Read the model definition and answer for the solid it produces. Units are mm, in the model's axes. A direction names the side the tool comes from. Coordinates: 2 decimals unless noted, no trailing zeros. Write each loop counter-clockwise with the first axis right and the second up, starting at its lowest first coordinate (ties: lowest second). Pieces come first, ordered by that corner, then holes.
1) Which of the six approach directions +Z, -Z, +X, -X, +Y, -Y give full straight-line access (tool end or side, diameter ignored) to faces 1 (the face through (23.368, 18, 0)), 2 (the face through (-18, 23.368, 18)), 3 (the face through (19.8, 9.6, -20.51)), 4 (the face through (15.174, 18.139, -14.999))?
2) The part is cut by section A-A (y = 9.5). Determine the outline of the cut face in (x, z), then the cut area to 3 significant figures.
3) Each of these flat-tipped pins is pushed along its axis until it touches: pin 1 Ø2 at (x, z) = (16, -19.5) entering from -Y; pin 2 Ø3.5 at (x, y) = (27.5, 22.5) entering from -Z; pin 3 Ø2 at (y, z) = (17.5, 13) entering from +X. Where does it stop, or does it pass through?
4) The part is cut by section C-C (y = 18). Determine the outline of the cut face in (x, z).
5) Find the intervals of material crossed by line 1 (Y direction, x = 1.5, z = 17.5) (3 decimals); line 2 (X direction, y = 30, z = -8.5); line 3 (Y direction, x = -20.5, z = -3.5) (3 decimals), in increasing order.
6) The part is cut by section B-B (z = 0). Determine the outline of the cut face in (x, y) (3 decimals), then the cut area to 3 significant figures.
7) The part is cut by section D-D (x = 7.5). Determine the outline of the cut face in (y, z) (3 decimals).
8) Determine the mould class of faces 5 (the face through (16, 20.32, -17.3)), 6 (the face through (-16.62, 8.52, 16.43)), 7 (the face through (16.34, 12.81, -18.98)) for opening direction X: +X half, -X half, draft (parallel to the pull), parting line (faces both ways), or undercut.
from build123d import *

# Parameters (mm, degrees)
BOSS_EXTRUDE1_DEPTH  = 35.56
SHELL1_T             = -2.032
SKETCH2_R            = 15.24
BOSS_EXTRUDE2_DEPTH  = 3.175
SKETCH3_R            = 4.064
BOSS_EXTRUDE3_DEPTH  = 2.8575
FILLET2_R            = 2.54
SKETCH4_R            = 4.064
BOSS_EXTRUDE10_DEPTH = 2.8575
BOSS_EXTRUDE11_DEPTH = 8.636
FILLET3_R            = 2.54
BOSS_EXTRUDE12_DEPTH = 46.736
SKETCH8_W            = 5.08
SKETCH8_H            = 22.86
CUT_EXTRUDE1_DEPTH   = 55.98528445


with BuildPart() as part:
    # Sketch1 → Boss-Extrude1 (new body)
    with BuildSketch(Plane(origin=(0, 0, 0), x_dir=(1, 0, 0), z_dir=(0, 1, 0))):
        Polygon((9.679342526, -23.368), (23.368, -9.679342526), (23.368, 9.679342526), (9.679342526, 23.368), (-9.679342526, 23.368), (-23.368, 9.679342526), (-23.368, -9.679342526), (-9.679342526, -23.368), align=None)
    extrude(amount=BOSS_EXTRUDE1_DEPTH)

    # Shell1
    shell1_openings = [part.faces().sort_by_distance(p)[0] for p in [
        (0, 0, 0),
    ]]
    offset(amount=SHELL1_T, openings=shell1_openings, kind=Kind.INTERSECTION)

    # Sketch2 → Boss-Extrude2 (add)
    with BuildSketch(Plane.XZ):
        Polygon((23.368, 9.679342526), (9.679342526, 23.368), (-9.679342526, 23.368), (-23.368, 9.679342526), (-23.368, -9.679342526), (-9.679342526, -23.368), (9.679342526, -23.368), (23.368, -9.679342526), align=None)
        with Locations(Location((0, 0, 0), (0, 0, 270))):
            Circle(SKETCH2_R, mode=Mode.SUBTRACT)
    extrude(amount=-BOSS_EXTRUDE2_DEPTH)

    # Sketch3 → Boss-Extrude3 (add)
    with BuildSketch(Plane(origin=(0, 0, -23.368), x_dir=(-1, 0, 0), z_dir=(0, 0, -1))):
        with BuildLine():
            Line((-9.679342526, 5.08), (-27.205342526, 5.08))
            ThreePointArc((-27.205342526, 5.08), (-34.825342526, 12.7), (-27.205342526, 20.32))
            Line((-27.205342526, 20.32), (-9.679342526, 20.32))
            Line((-9.679342526, 20.32), (-9.679342526, 5.08))
        make_face()
        with Locations((-27.205342526, 12.7)):
            Circle(SKETCH3_R, mode=Mode.SUBTRACT)
    extrude(amount=-BOSS_EXTRUDE3_DEPTH)

    # Fillet2
    fillet2_edges = [part.edges().sort_by_distance(p)[0] for p in [
        (12.536842526, 12.7, -20.5105),
    ]]
    fillet(fillet2_edges, radius=FILLET2_R)

    # Sketch4 → Boss-Extrude10 (add)
    with BuildSketch(Plane.XY.offset(-20.5105)):
        with BuildLine():
            Line((12.981342526, 19.304), (12.981342526, 29.464))
            Line((12.981342526, 29.464), (24.665342526, 29.464))
            Line((24.665342526, 29.464), (33.422629122, 17.105649484))
            ThreePointArc((33.422629122, 17.105649484), (29.517124969, 5.439141791), (19.585342526, 12.7))
            Line((19.585342526, 12.7), (19.585342526, 19.304))
            Line((19.585342526, 19.304), (12.981342526, 19.304))
        make_face()
        with Locations(Location((27.205342526, 12.7, 0), (0, 0, 180))):
            Circle(SKETCH4_R, mode=Mode.SUBTRACT)
    extrude(amount=BOSS_EXTRUDE10_DEPTH)

    # Sketch5 → Boss-Extrude11 (add)
    with BuildSketch(Plane(origin=(0, 29.464, 0), x_dir=(1, 0, 0), z_dir=(0, 1, 0))):
        Polygon((12.536842526, 20.5105), (21.934842526, 20.5105), (21.934842526, 11.1125), align=None)
    extrude(amount=-BOSS_EXTRUDE11_DEPTH)

    # Fillet3
    fillet3_edges = [part.edges().sort_by_distance(p)[0] for p in [
        (21.934842526, 25.146, -17.653),
    ]]
    fillet(fillet3_edges, radius=FILLET3_R)

    # Sketch6 → Boss-Extrude12 (add, through all)
    with BuildSketch(Plane.XY.offset(23.368)):
        with BuildLine():
            Line((-9.679342526, 17.272), (-23.141342526, 17.272))
            ThreePointArc((-23.141342526, 17.272), (-26.189342526, 20.32), (-23.141342526, 23.368))
            Line((-23.141342526, 23.368), (-9.679342526, 23.368))
            Line((-9.679342526, 23.368), (-9.679342526, 17.272))
        make_face()
    extrude(amount=-BOSS_EXTRUDE12_DEPTH)

    # Sketch8 → Cut-Extrude1 (cut, through all)
    with BuildSketch(Plane(origin=(0, 35.56, 0), x_dir=(1, 0, 0), z_dir=(0, 1, 0))):
        with Locations((-25.908, 0)):
            Rectangle(SKETCH8_W, SKETCH8_H)
    extrude(amount=-CUT_EXTRUDE1_DEPTH, mode=Mode.SUBTRACT)


solid = part.part
Reported:
1. face 1: +Z, +X, +Y, -Y
1. face 2: +Z, -X, +Y
1. face 3: -Y
1. face 4: none
2. outline: (-23.37, -9.68) - (-9.68, -23.37) - (24.7, -23.37) - (24.7, -17.65) - (20.29, -17.65) - (20.29, -20.51) - (18.67, -20.51) arc R2.54 cw to (16.87, -16.17) - (23.37, -9.68) - (23.37, 9.68) - (9.68, 23.37) - (-9.68, 23.37) - (-23.37, 9.68) - close; (29.71, -23.37) - (34.12, -23.37) - (34.12, -17.65) - (29.71, -17.65) - close; hole (-21.34, -8.84) - (-8.84, -21.34) - (8.84, -21.34) - (21.34, -8.84) - (21.34, 8.84) - (8.84, 21.34) - (-8.84, 21.34) - (-21.34, 8.84) - close
2. area: 386 mm2
3. pin 1: stops at y = 5.08
3. pin 2: stops at z = -20.51
3. pin 3: stops at x = 21.05
4. outline: (-25.12, -23.37) - (32.68, -23.37) - (32.68, -20.51) - (32.79, -20.51) - (32.79, -17.65) - (19.59, -17.65) - (19.59, -20.51) - (18.67, -20.51) arc R2.54 cw to (16.87, -16.17) - (23.37, -9.68) - (23.37, 9.68) - (9.68, 23.37) - (-25.12, 23.37) - (-25.12, 11.43) - (-23.37, 11.43) - (-23.37, -11.43) - (-25.12, -11.43) - close; hole (-9.68, -20.49) - (-8.84, -21.34) - (8.84, -21.34) - (21.34, -8.84) - (21.34, 8.84) - (8.84, 21.34) - (-8.84, 21.34) - (-9.68, 20.49) - close
5. line 1: y = 0 to 3.175, 33.528 to 35.56
5. line 2: x = -23.37 to -21.34, 21.34 to 23.37
5. line 3: y = 0 to 3.175, 17.272 to 23.368, 33.528 to 35.56
6. outline: (-23.368, 0) - (-15.24, 0) - (-15.24, 3.175) - (-21.336, 3.175) - (-21.336, 17.272) - (-9.679, 17.272) - (-9.679, 23.368) - (-21.336, 23.368) - (-21.336, 33.528) - (21.336, 33.528) - (21.336, 3.175) - (15.24, 3.175) - (15.24, 0) - (23.368, 0) - (23.368, 35.56) - (-23.368, 35.56) - close
6. area: 341 mm2
7. outline: (0, -23.368) - (35.56, -23.368) - (35.56, 23.368) - (0, 23.368) - (0, 13.267) - (3.175, 13.267) - (3.175, 21.336) - (33.528, 21.336) - (33.528, -21.336) - (3.175, -21.336) - (3.175, -13.267) - (0, -13.267) - close
8. face 5: draft
8. face 6: -X half
8. face 7: undercut
